For this review, use the dimensioned drawing (mm, ordinates from the lowest corner) and the shaded views. Coordinates: 2 decimals unless noted, no trailing zeros. Write each loop counter-clockwise with the first axis right and the second up, starting at its lowest first coordinate (ties: lowest second). Pieces come first, ordered by that corner, then holes. Notation, with made-up numbers: M -5,-11 L 41,-11 A13 ccw 41,7 Z; hole C 83.25,-14.5 d8. An arc over 180 degrees is marked long. One line per question, with ' | ' between items.
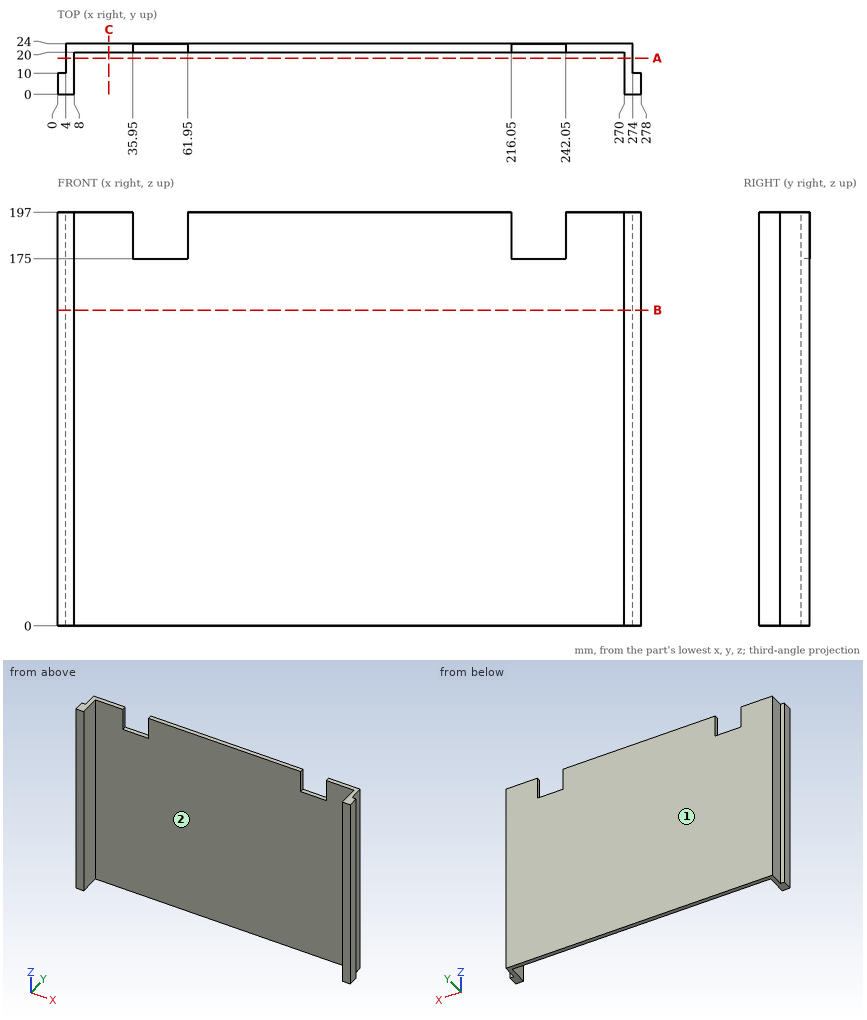
1) We need section A-A on y = 17.25. State the section outline as (x, z) points.
Responses:
outline: M 4,0 L 8,0 L 8,197 L 4,197 Z; M 270,0 L 274,0 L 274,197 L 270,197 Z
2) We need section C-C on x = 24.5. State the section outline as (y, z) points, then the cut area to 3 significant figures.
Responses:
outline: M 20,0 L 24,0 L 24,197 L 20,197 Z | area: 788 mm^2
3) The part is to be moulded in two halves that separate along X. For the marked faces 1 and 2, say which applies: +X half, -X half, draft (parallel to the pull), parting line (faces both ways), or undercut.
Responses:
face 1: draft | face 2: undercut
4) We need section B-B on z = 150.5. State the section outline as (x, y) points, then the cut area to 3 significant figures.
Responses:
outline: M 0,0 L 8,0 L 8,20 L 270,20 L 270,0 L 278,0 L 278,10 L 274,10 L 274,24 L 4,24 L 4,10 L 0,10 Z | area: 1,320 mm^2
5) To check wall thickness, follow line 1 along X through (y, z) = (12.5, 83.5); line 2 along X through (y, z) = (8.5, 117); line 3 along Y through (x, z) = (217, 22). State the ranges of each line that lie inside material, in increasing order. Write a range as [from, to].
Responses:
line 1: [4, 8], [270, 274] | line 2: [0, 8], [270, 278] | line 3: [20, 24]
6) Insertion check: pin 1 Ø4.5 at (y, z) = (23, 183) entering from +X; pin 2 Ø1.2 at (x, z) = (276.5, 95.5) entering from +Y; pin 3 Ø6 at (x, z) = (48, 121) entering from -Y; pin 4 Ø12 at (x, y) = (52.5, 13.5) entering from +Z. Each pin has a flat end and moves straight along its axis. Give the tip position at first contact, or say it passes through.
Responses:
pin 1: x = 274 | pin 2: y = 10 | pin 3: y = 20 | pin 4: through
